Geometry check sheet. Reference: the model listing, model coordinates, mm. Give positions to 0.01 mm unless a question says otherwise; leave off trailing zeros. Order: outer loops, then holes, each group sorted by start corner. A loop starts at its lowest first (then second) coordinate and runs counter-clockwise, first axis right, second up. Notation, with made-up numbers: M 17,67 L 60,67 A29 cw 60,105 Z; hole C 68.25,-32 d5. An arc over 180 degrees is marked long. Put each result on its own line as item: value. Start each with the question number.
Q1. Section check B-B on y = 0. Record the cut outline in (x, z).
Q2. Section check D-D on x = -5. Record the cut outline in (y, z) (3 decimals).
Q3. Go/stop test with a flat-tipped pin: pin 1 (11 mm diameter, centred on x = 0, y = 0, fed in from +Z). Record where the tip stops, or that it passes through.
Q4. Section check C-C on z = 0.05. State how many separate pieces and enclosed holes the cut face has, then the cut area to 3 significant figures.
Q5. Material ranges on L1, parallel to X at y = 11.75, z = 0.1; L2, parallel to X at y = 13.25, z = 0.1; L3, parallel to Y at x = 7, z = 0.05, recorded low to high.
Q6. Section check A-A on x = 0. Record the cut outline in (y, z), then the cut area to 3 significant figures.
```python
from build123d import *

# Parameters (mm, degrees)
F0_R     = 0.45
F0_R_2   = 6
F1_DEPTH = 0.14


with BuildPart() as f1:
    # F0 (on Top) → F1 (new body)
    with BuildSketch(Plane.XY):
        with BuildLine():
            ThreePointArc((7.964766, -0.75), (7.991187, -0.375414), (8, 0))
            ThreePointArc((8, 0), (7.991187, 0.375414), (7.964766, 0.75))
            ThreePointArc((7.964766, 0.75), (7.727407, 2.070552), (7.27269, 3.332864))
            ThreePointArc((7.27269, 3.332864), (6.928203, 4), (6.52269, 4.631902))
            ThreePointArc((6.52269, 4.631902), (6.128356, 5.142301), (5.694186, 5.619274))
            ThreePointArc((5.694186, 5.619274), (5.142301, 6.128356), (4.54512, 6.583456))
            ThreePointArc((4.54512, 6.583456), (4, 6.928203), (3.42888, 7.227917))
            ThreePointArc((3.42888, 7.227917), (2.736161, 7.517541), (2.019341, 7.740947))
            ThreePointArc((2.019341, 7.740947), (1.389185, 7.878462), (0.75, 7.964766))
            ThreePointArc((0.75, 7.964766), (0, 8), (-0.75, 7.964766))
            ThreePointArc((-0.75, 7.964766), (-1.389185, 7.878462), (-2.019341, 7.740947))
            ThreePointArc((-2.019341, 7.740947), (-2.736161, 7.517541), (-3.42888, 7.227917))
            ThreePointArc((-3.42888, 7.227917), (-4, 6.928203), (-4.54512, 6.583456))
            ThreePointArc((-4.54512, 6.583456), (-5.142301, 6.128356), (-5.694186, 5.619274))
            ThreePointArc((-5.694186, 5.619274), (-6.553216, 4.588611), (-7.227917, 3.42888))
            ThreePointArc((-7.227917, 3.42888), (-7.517541, 2.736161), (-7.740947, 2.019341))
            ThreePointArc((-7.740947, 2.019341), (-7.878462, 1.389185), (-7.964766, 0.75))
            ThreePointArc((-7.964766, 0.75), (-8, 0), (-7.964766, -0.75))
            ThreePointArc((-7.964766, -0.75), (-7.878462, -1.389185), (-7.740947, -2.019341))
            ThreePointArc((-7.740947, -2.019341), (-7.517541, -2.736161), (-7.227917, -3.42888))
            ThreePointArc((-7.227917, -3.42888), (-6.928203, -4), (-6.583456, -4.54512))
            ThreePointArc((-6.583456, -4.54512), (-6.128356, -5.142301), (-5.619274, -5.694186))
            ThreePointArc((-5.619274, -5.694186), (-5.142301, -6.128356), (-4.631902, -6.52269))
            ThreePointArc((-4.631902, -6.52269), (-4, -6.928203), (-3.332864, -7.27269))
            ThreePointArc((-3.332864, -7.27269), (-2.736161, -7.517541), (-2.121673, -7.713527))
            ThreePointArc((-2.121673, -7.713527), (-1.389185, -7.878462), (-0.644461, -7.974))
            ThreePointArc((-0.644461, -7.974), (0, -8), (0.644461, -7.974))
            ThreePointArc((0.644461, -7.974), (1.389185, -7.878462), (2.121673, -7.713527))
            ThreePointArc((2.121673, -7.713527), (2.736161, -7.517541), (3.332864, -7.27269))
            ThreePointArc((3.332864, -7.27269), (4, -6.928203), (4.631902, -6.52269))
            ThreePointArc((4.631902, -6.52269), (5.142301, -6.128356), (5.619274, -5.694186))
            ThreePointArc((5.619274, -5.694186), (6.128356, -5.142301), (6.583456, -4.54512))
            ThreePointArc((6.583456, -4.54512), (6.928203, -4), (7.227917, -3.42888))
            ThreePointArc((7.227917, -3.42888), (7.517541, -2.736161), (7.740947, -2.019341))
            ThreePointArc((7.740947, -2.019341), (7.878462, -1.389185), (7.964766, -0.75))
        make_face()
        with Locations((-7, 0)):
            Circle(F0_R, mode=Mode.SUBTRACT)
        Circle(F0_R_2, mode=Mode.SUBTRACT)
        with Locations((7, 0)):
            Circle(F0_R, mode=Mode.SUBTRACT)
        with BuildLine():
            ThreePointArc((7.964766, 0.75), (7.991187, 0.375414), (8, 0))
            ThreePointArc((8, 0), (7.991187, -0.375414), (7.964766, -0.75))
            Line((7.964766, -0.75), (14.25, -0.75))
            ThreePointArc((14.25, -0.75), (15, 0), (14.25, 0.75))
            Line((14.25, 0.75), (7.964766, 0.75))
        make_face()
        with BuildLine():
            ThreePointArc((6.52269, 4.631902), (6.928203, 4), (7.27269, 3.332864))
            Line((7.27269, 3.332864), (12.715862, 6.475481))
            ThreePointArc((12.715862, 6.475481), (12.990381, 7.5), (11.965862, 7.774519))
            Line((11.965862, 7.774519), (6.52269, 4.631902))
        make_face()
        with BuildLine():
            Line((13.647135, -4.169018), (7.740947, -2.019341))
            ThreePointArc((7.740947, -2.019341), (7.517541, -2.736161), (7.227917, -3.42888))
            Line((7.227917, -3.42888), (13.134105, -5.578557))
            ThreePointArc((13.134105, -5.578557), (14.095389, -5.130302), (13.647135, -4.169018))
        make_face()
        with BuildLine():
            ThreePointArc((4.54512, 6.583456), (5.142301, 6.128356), (5.694186, 5.619274))
            Line((5.694186, 5.619274), (9.734257, 10.434043))
            ThreePointArc((9.734257, 10.434043), (9.641814, 11.490667), (8.58519, 11.398224))
            Line((8.58519, 11.398224), (4.54512, 6.583456))
        make_face()
        with BuildLine():
            Line((11.398224, -8.58519), (6.583456, -4.54512))
            ThreePointArc((6.583456, -4.54512), (6.128356, -5.142301), (5.619274, -5.694186))
            Line((5.619274, -5.694186), (10.434043, -9.734257))
            ThreePointArc((10.434043, -9.734257), (11.490667, -9.641814), (11.398224, -8.58519))
        make_face()
        with BuildLine():
            ThreePointArc((2.019341, 7.740947), (2.736161, 7.517541), (3.42888, 7.227917))
            Line((3.42888, 7.227917), (5.578557, 13.134105))
            ThreePointArc((5.578557, 13.134105), (5.130302, 14.095389), (4.169018, 13.647135))
            Line((4.169018, 13.647135), (2.019341, 7.740947))
        make_face()
        with BuildLine():
            Line((7.774519, -11.965862), (4.631902, -6.52269))
            ThreePointArc((4.631902, -6.52269), (4, -6.928203), (3.332864, -7.27269))
            Line((3.332864, -7.27269), (6.475481, -12.715862))
            ThreePointArc((6.475481, -12.715862), (7.5, -12.990381), (7.774519, -11.965862))
        make_face()
        with BuildLine():
            ThreePointArc((-0.75, 7.964766), (0, 8), (0.75, 7.964766))
            Line((0.75, 7.964766), (0.75, 14.25))
            ThreePointArc((0.75, 14.25), (0, 15), (-0.75, 14.25))
            Line((-0.75, 14.25), (-0.75, 7.964766))
        make_face()
        with BuildLine():
            Line((3.213092, -13.903274), (2.121673, -7.713527))
            ThreePointArc((2.121673, -7.713527), (1.389185, -7.878462), (0.644461, -7.974))
            Line((0.644461, -7.974), (1.735881, -14.163747))
            ThreePointArc((1.735881, -14.163747), (2.604723, -14.772116), (3.213092, -13.903274))
        make_face()
        with BuildLine():
            ThreePointArc((-3.42888, 7.227917), (-2.736161, 7.517541), (-2.019341, 7.740947))
            Line((-2.019341, 7.740947), (-4.169018, 13.647135))
            ThreePointArc((-4.169018, 13.647135), (-5.130302, 14.095389), (-5.578557, 13.134105))
            Line((-5.578557, 13.134105), (-3.42888, 7.227917))
        make_face()
        with BuildLine():
            Line((-1.735881, -14.163747), (-0.644461, -7.974))
            ThreePointArc((-0.644461, -7.974), (-1.389185, -7.878462), (-2.121673, -7.713527))
            Line((-2.121673, -7.713527), (-3.213092, -13.903274))
            ThreePointArc((-3.213092, -13.903274), (-2.604723, -14.772116), (-1.735881, -14.163747))
        make_face()
        with BuildLine():
            ThreePointArc((-5.694186, 5.619274), (-5.142301, 6.128356), (-4.54512, 6.583456))
            Line((-4.54512, 6.583456), (-8.58519, 11.398224))
            ThreePointArc((-8.58519, 11.398224), (-9.641814, 11.490667), (-9.734257, 10.434043))
            Line((-9.734257, 10.434043), (-5.694186, 5.619274))
        make_face()
        with BuildLine():
            Line((-6.475481, -12.715862), (-3.332864, -7.27269))
            ThreePointArc((-3.332864, -7.27269), (-4, -6.928203), (-4.631902, -6.52269))
            Line((-4.631902, -6.52269), (-7.774519, -11.965862))
            ThreePointArc((-7.774519, -11.965862), (-7.5, -12.990381), (-6.475481, -12.715862))
        make_face()
        with BuildLine():
            ThreePointArc((-7.740947, 2.019341), (-7.517541, 2.736161), (-7.227917, 3.42888))
            Line((-7.227917, 3.42888), (-13.134105, 5.578557))
            ThreePointArc((-13.134105, 5.578557), (-14.095389, 5.130302), (-13.647135, 4.169018))
            Line((-13.647135, 4.169018), (-7.740947, 2.019341))
        make_face()
        with BuildLine():
            Line((-10.434043, -9.734257), (-5.619274, -5.694186))
            ThreePointArc((-5.619274, -5.694186), (-6.128356, -5.142301), (-6.583456, -4.54512))
            Line((-6.583456, -4.54512), (-11.398224, -8.58519))
            ThreePointArc((-11.398224, -8.58519), (-11.490667, -9.641814), (-10.434043, -9.734257))
        make_face()
        with BuildLine():
            ThreePointArc((-7.964766, -0.75), (-8, 0), (-7.964766, 0.75))
            Line((-7.964766, 0.75), (-14.25, 0.75))
            ThreePointArc((-14.25, 0.75), (-15, 0), (-14.25, -0.75))
            Line((-14.25, -0.75), (-7.964766, -0.75))
        make_face()
        with BuildLine():
            Line((-13.134105, -5.578557), (-7.227917, -3.42888))
            ThreePointArc((-7.227917, -3.42888), (-7.517541, -2.736161), (-7.740947, -2.019341))
            Line((-7.740947, -2.019341), (-13.647135, -4.169018))
            ThreePointArc((-13.647135, -4.169018), (-14.095389, -5.130302), (-13.134105, -5.578557))
        make_face()
    extrude(amount=F1_DEPTH)


solid = f1.part
```
Results found:
1. outline: M -15,0 L -7.45,0 L -7.45,0.14 L -15,0.14 Z; M -6.55,0 L -6,0 L -6,0.14 L -6.55,0.14 Z; M 6,0 L 6.55,0 L 6.55,0.14 L 6,0.14 Z; M 7.45,0 L 15,0 L 15,0.14 L 7.45,0.14 Z
2. outline: M -10.16,0 L -7.16,0 L -7.16,0.14 L -10.16,0.14 Z; M -6.245,0 L -3.317,0 L -3.317,0.14 L -6.245,0.14 Z; M 3.317,0 L 7.126,0 L 7.126,0.14 L 3.317,0.14 Z; M 11.545,0 L 14.13,0 L 14.13,0.14 L 11.545,0.14 Z
3. pin 1: passes through
4. separate pieces: 1
4. enclosed holes: 3
4. area: 261 mm^2
5. L1: x = -5.07 to -3.48, -0.75 to 0.75, 3.48 to 5.07
5. L2: x = -5.61 to -4.02, -0.75 to 0.75, 4.02 to 5.61
5. L3: y = -13.08 to -10.62, -6.85 to -4.89, -3.87 to -0.45, 0.45 to 4.91, 7.18 to 9.51
6. outline: M -8,0 L -6,0 L -6,0.14 L -8,0.14 Z; M 6,0 L 15,0 L 15,0.14 L 6,0.14 Z
6. area: 1.54 mm^2
